Input: part model. Units: mm. Frame: model coordinates. Coordinates: 2 decimals unless noted, no trailing zeros. Write each loop counter-clockwise with the first axis right and the second up, starting at its lowest first coordinate (ties: lowest second). Pieces come first, ordered by that corner, then holes. Notation, with made-up numbers: M 33.5,22.25 L 46.5,22.25 A7 ccw 46.5,35.25 Z; hole C 72,-35.5 d10. An arc over 180 degrees is marked long. Use one line per item in the form item = value.
from build123d import *

# Parameters (mm, degrees)
F0_W     = 10
F0_H     = 10
F1_DEPTH = 20
F2_W     = 2
F2_H     = 10
F2_W_2   = 10
F3_DEPTH = 10
F6_R     = 4.99999
F5_W     = 10
F5_H     = 10
F5_R     = 3
F7_DEPTH = 2
F4_W     = 10
F4_H     = 10
F4_R     = 3
F8_DEPTH = 2
F9_DEPTH = 14.001


# Not quite as in the source:
# - a fillet or chamfer is up to 0.001 mm smaller than in the source, because OpenCascade refuses the exact size


with BuildPart() as f1:
    # F0 (on Top) → F1 (new body)
    with BuildSketch(Plane.XY):
        Rectangle(F0_W, F0_H)
    extrude(amount=F1_DEPTH)

    # F2 (on face) → F3 (join)
    with BuildSketch(Plane.XY.offset(20)):
        with Locations((-6, 0)):
            Rectangle(F2_W, F2_H)
        Rectangle(F2_W_2, F2_H)
        with Locations((6, 0)):
            Rectangle(F2_W, F2_H)
    extrude(amount=F3_DEPTH)

    # F6 (radius 5 in the source; OpenCascade refuses exactly that, so slightly less here)
    f6_edges = [f1.edges().sort_by_distance(p)[0] for p in [
        (0, 5, 30),
        (0, -5, 30),
    ]]
    fillet(f6_edges, radius=F6_R)

    # F5 (on face) → F7 (cut)
    with BuildSketch(Plane.YZ.offset(7)):
        with Locations((0, 25)):
            Rectangle(F5_W, F5_H)
        with Locations((0, 25)):
            Circle(F5_R, mode=Mode.SUBTRACT)
    extrude(amount=-F7_DEPTH, mode=Mode.SUBTRACT)

    # F4 (on face) → F8 (cut)
    with BuildSketch(Plane(origin=(-7, 0, 0), x_dir=(0, -1, 0), z_dir=(-1, 0, 0))):
        with Locations((0, 25)):
            Rectangle(F4_W, F4_H)
        with Locations((0, 25)):
            Circle(F4_R, mode=Mode.SUBTRACT)
    extrude(amount=-F8_DEPTH, mode=Mode.SUBTRACT)

    # F9 (cut, through all): a face of the model
    f9_faces = [f1.faces().sort_by_distance(p)[0] for p in [
        (-7, 0, 25),
    ]]
    extrude(f9_faces, amount=-F9_DEPTH, mode=Mode.SUBTRACT)


solid = f1.part
(1) Section query C-C on z = 23. Return the cut outline in (x, y), plus the area to 3 significant figures.
Computed:
outline = M -5,-5 L 5,-5 L 5,-2.24 L -5,-2.24 Z; M -5,2.24 L 5,2.24 L 5,5 L -5,5 Z
area = 55.3 mm^2
(2) First-contact query: pin 1 Ø2 at (x, y) = (-3, 1) entering from -Z. Flat tip, straight axial feed; report the tip coordinate or a pass-through.
Computed:
pin_1 = 0
(3) Line query: probe 1 along Z at (x, y) = (-1.75, 0); probe 2 along Y at (x, z) = (-2.75, 25); probe 3 along Y at (x, z) = (-4.25, 26.75). Output: solid intervals per line, ascending.
Computed:
probe_1 = 0 to 22, 28 to 30
probe_2 = -5 to -3, 3 to 5
probe_3 = -4.68 to -2.44, 2.44 to 4.68
(4) Section query B-B on y = -2.5. Return the cut outline in (x, z), plus the area to 3 significant figures.
Computed:
outline = M -5,0 L 5,0 L 5,23.34 L -5,23.34 Z; M -5,26.66 L 5,26.66 L 5,29.33 L -5,29.33 Z
area = 260 mm^2
(5) Pull-direction query (Z, two-part tool) for faces 1 (the cylindrical face through (-0.07, 0.65, 22.07)), 2 (the flat face through (0, 0, 0)), 3 (the cylindrical face through (0, 4, 28)), 4 (the flat face through (0, 5, 12)); classes: pulls with the +Z half, pulls with the -Z half, needs draft (parallel to the pull), parting line crosses it, or undercut.
Computed:
face_1 = undercut
face_2 = pulls with the -Z half
face_3 = pulls with the +Z half
face_4 = needs draft
